from build123d import *

# Parameters (mm, degrees)
SKETCH1_R           = 3.25
BOSS_EXTRUDE1_DEPTH = 2.5
SKETCH2_R           = 5.25
BOSS_EXTRUDE2_DEPTH = 1


with BuildPart() as part:
    # Sketch1 → Boss-Extrude1 (new, symmetric)
    with BuildSketch(Plane.XY):
        Circle(SKETCH1_R)
        Polygon((3.117691454, 0), (1.558845727, 2.7), (-1.558845727, 2.7), (-3.117691454, 0), (-1.558845727, -2.7), (1.558845727, -2.7), align=None, mode=Mode.SUBTRACT)
    extrude(amount=BOSS_EXTRUDE1_DEPTH, both=True)

    # Sketch2 → Boss-Extrude2 (add)
    with BuildSketch(Plane.XY.offset(2.5)):
        Circle(SKETCH2_R)
        Polygon((3.117691454, 0), (1.558845727, 2.7), (-1.558845727, 2.7), (-3.117691454, 0), (-1.558845727, -2.7), (1.558845727, -2.7), align=None, mode=Mode.SUBTRACT)
    extrude(amount=BOSS_EXTRUDE2_DEPTH)


solid = part.part
Design review of the part built by this model. Coordinates are the model's own, in mm. A direction names the side the tool comes from. Coordinates: 2 decimals unless noted, no trailing zeros. Order: outer loops, then holes, each group sorted by start corner. A loop starts at its lowest first (then second) coordinate and runs counter-clockwise, first axis right, second up. Notation, with made-up numbers: (-5.75, 73.25) - (24.25, 73.25) arc R23 ccw to (24.25, 96.25) - close; hole circle Ø1 at (82, 28). An arc over 180 degrees is marked (long way). Put each result on its own line as item: value.
1) The part is to be moulded in two halves that separate along Y. For faces 3 (the face through (-2.327, 1.369, 0.458)), 4 (the face through (-0.1, -3.4, 2.5)), 5 (the face through (-2.579, -1.978, 0.035)), say which applies: released by +Y, released by -Y, zero draft, split by the parting line, or undercut.
Response values:
face 3: undercut
face 4: zero draft
face 5: split by the parting line
2) Tool access review of faces 1 (the face through (0, 2.7, 0)), 2 (the face through (2.3, -2.3, 3.5)): name each direction out of +Z, -Z, +X, -X, +Y, -Y from which nothing blocks a thin tool from reaching the whole face with its end or side.
Response values:
face 1: +Z, -Z
face 2: +Z, +X, -X, +Y, -Y
3) Insertion check: P1, Ø0.9, axis at x = 0, z = 0, coming from the -Y side; P2, Ø2.5, axis at x = -0.5, z = 1, coming from the +Y side; P3, Ø3, axis at x = -0.5, y = 1, coming from the -Z side; P4, Ø1, axis at x = 3.5, y = -3.5, coming from the -Z side. Each pin has a flat end and moves straight along its axis. Give the tip position at first contact, or say it passes through.
Response values:
P1: stops at y = -3.25
P2: stops at y = 3.25
P3: passes through
P4: stops at z = 2.5
4) Wall thickness on L1, parallel to Z at x = 1.25, y = 4; L2, parallel to Y at x = 0, z = 2.15; L3, parallel to Y at x = 1.75, z = 0.4: over which ranges is each line inside the solid? List them lowest first. Write a range as from..to.
Response values:
L1: z = 2.5..3.5
L2: y = -3.25..-2.7, 2.7..3.25
L3: y = -2.74..-2.37, 2.37..2.74
5) Take a section at B-B, the plane z = 0.9. Give the boundary of the cut face in (x, y), and give its area (3 significant figures).
Response values:
outline: circle Ø6.5 at (0, 0); hole (-3.12, 0) - (-1.56, -2.7) - (1.56, -2.7) - (3.12, 0) - (1.56, 2.7) - (-1.56, 2.7) - close
area: 7.93 mm²
6) Take a section at A-A, the plane y = -0.25. Give the boundary of the cut face in (x, z), and give its area (3 significant figures).
Response values:
outline: (-5.24, 2.5) - (-3.24, 2.5) - (-3.24, -2.5) - (-2.97, -2.5) - (-2.97, 3.5) - (-5.24, 3.5) - close; (2.97, -2.5) - (3.24, -2.5) - (3.24, 2.5) - (5.24, 2.5) - (5.24, 3.5) - (2.97, 3.5) - close
area: 7.21 mm²
7) Take a section at C-C, the plane x = 0. Give the boundary of the cut face in (y, z), and give its area (3 significant figures).
Response values:
outline: (-5.25, 2.5) - (-3.25, 2.5) - (-3.25, -2.5) - (-2.7, -2.5) - (-2.7, 3.5) - (-5.25, 3.5) - close; (2.7, -2.5) - (3.25, -2.5) - (3.25, 2.5) - (5.25, 2.5) - (5.25, 3.5) - (2.7, 3.5) - close
area: 10.6 mm²
8) Take a section at D-D, the plane y = 4.25. Give the boundary of the cut face in (x, z), and give its area (3 significant figures).
Response values:
outline: (-3.08, 2.5) - (3.08, 2.5) - (3.08, 3.5) - (-3.08, 3.5) - close
area: 6.16 mm²
